Can you work these out from the model? Positions are in its coordinate system, mm. Give positions to 0.01 mm unless a question says otherwise; leave off trailing zeros. Write each loop counter-clockwise with the first axis right and the second up, starting at its lowest first coordinate (ties: lowest second). Pieces come first, ordered by that corner, then holes. Notation, with made-up numbers: (-30, -3) - (-2, -3) arc R14 cw to (-2, 8) - close; hole circle Ø6 at (81, 64). An arc over 180 degrees is marked (long way). Use a Markdown table: item, result. Add a question column.
```python
from build123d import *

# Parameters (mm, degrees)
F1_DEPTH      = 14
F1_DEPTH_BACK = 14
F2_R          = 10.5


with BuildPart() as f1:
    # F0 (on Front) → F1 (new body, two sides)
    with BuildSketch(Plane.XZ) as f1_sk:
        Polygon((5.135478, 10.66393), (-5.135478, 10.66393), (-11.539315, 2.633773), (-9.253812, -7.379669), (0, -11.83607), (9.253812, -7.379669), (11.539315, 2.633773), align=None)
    extrude(amount=F1_DEPTH)
    extrude(f1_sk.sketch, amount=-F1_DEPTH_BACK)

    # F2
    f2_edges = [f1.edges().sort_by_distance(p)[0] for p in [
        (-10.396563, -14, -2.372948),
        (-4.626906, -14, -9.607869),
        (4.626906, -14, -9.607869),
        (10.396563, -14, -2.372948),
        (8.337396, -14, 6.648852),
        (0, -14, 10.66393),
        (-8.337396, -14, 6.648852),
        (-10.396563, 14, -2.372948),
        (-4.626906, 14, -9.607869),
        (4.626906, 14, -9.607869),
        (10.396563, 14, -2.372948),
        (8.337396, 14, 6.648852),
        (0, 14, 10.66393),
        (-8.337396, 14, 6.648852),
    ]]
    fillet(f2_edges, radius=F2_R)


solid = f1.part
```
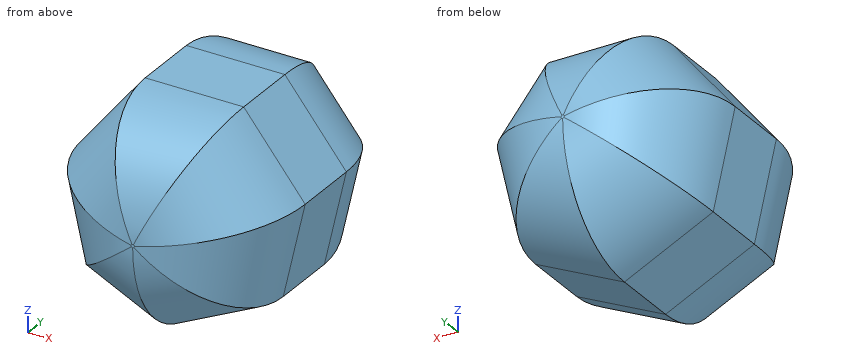
Q1. I'm going to push flat-ended pins straight in: P1, Ø4, axis at y = -4.5, z = 3.5, coming from the +X side; P2, Ø1.5, axis at x = -5.5, y = -3, coming from the -Z side; P3, Ø8, axis at x = 0, z = 5.5, coming from the -Y side; P4, Ø2, axis at x = -7, y = -4.5, coming from the +Z side. Where does each tip first touch, or does it pass through?
Q2. Suppose I cut it at B-B (y = -5). Please give me the cut outline in (x, z).
Q3. If I drill on probe 1 along X at (y, z) = (9, 3); probe 2 along Z at (x, y) = (-1, -6.75); probe 3 along X at (y, z) = (5.75, 0), over which ranges is the centre line in solid material (lowest first)? Write a range as [from, to].
Q4. Suppose I cut it at A-A (y = 0). Please give me the cut outline in (x, z).
Derived:
| question | item | result |
|---|---|---|
| 1 | P1 | x = 11.54 |
| 1 | P2 | z = -9.55 |
| 1 | P3 | y = -13.91 |
| 1 | P4 | z = 9.51 |
| 2 | outline | (-11.42, 2.61) - (-9.16, -7.31) - (0, -11.72) - (9.16, -7.31) - (11.42, 2.61) - (5.08, 10.56) - (-5.08, 10.56) - close |
| 3 | probe 1 | [-9.26, 9.26] |
| 3 | probe 2 | [-10.78, 10.15] |
| 3 | probe 3 | [-10.69, 10.69] |
| 4 | outline | (-11.54, 2.63) - (-9.25, -7.38) - (0, -11.84) - (9.25, -7.38) - (11.54, 2.63) - (5.14, 10.66) - (-5.14, 10.66) - close |
